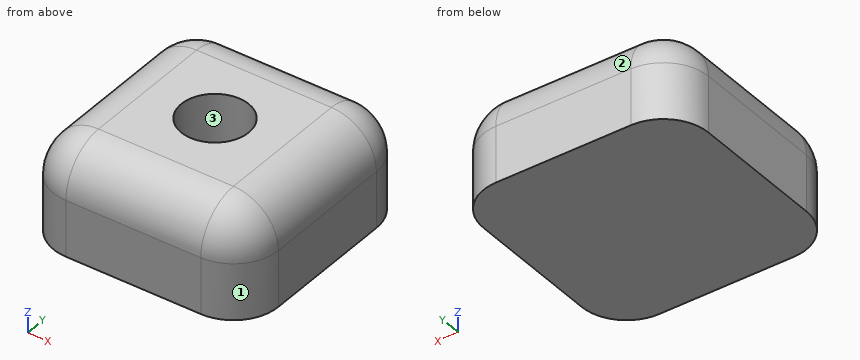
```python
from build123d import *

# Parameters (mm, degrees)
F0_W     = 25.4
F0_H     = 25.4
F1_DEPTH = 11.43
F2_R     = 3.81
F3_DEPTH = 6.35
F4_R     = 5.08


with BuildPart() as f1:
    # F0 (on Top) → F1 (new body)
    with BuildSketch(Plane.XY):
        with Locations((12.7, 12.7)):
            Rectangle(F0_W, F0_H)
    extrude(amount=F1_DEPTH)

    # F2 (on face) → F3 (cut)
    with BuildSketch(Plane.XY.offset(11.43)):
        with Locations((12.7, 12.7)):
            Circle(F2_R)
    extrude(amount=-F3_DEPTH, mode=Mode.SUBTRACT)

    # F4
    f4_edges = [f1.edges().sort_by_distance(p)[0] for p in [
        (25.4, 12.7, 11.43),
        (12.7, 25.4, 11.43),
        (0, 12.7, 11.43),
        (12.7, 0, 11.43),
        (25.4, 25.4, 5.715),
        (25.4, 0, 5.715),
        (0, 25.4, 5.715),
        (0, 0, 5.715),
    ]]
    fillet(f4_edges, radius=F4_R)


solid = f1.part
```
The listing builds one solid part. Answer for the finished solid, in the listing's coordinates (mm). Face numbers are marked on the shaded views. Coordinates: 2 decimals unless noted, no trailing zeros. Loops run counter-clockwise (first coordinate to the right, second up) from the corner with the lowest first, then second, coordinate; pieces in that order, holes last. Notation, with made-up numbers: (23.25, 31.25) -> (52.25, 31.25) arc R24 cw to (52.25, 62.25) -> close; hole circle Ø2 at (51.5, 63.5). An arc over 180 degrees is marked (long way). Use one line per item in the form item = value. Start each with the question number.
Item 1: The part is cut by section B-B on x = 12.7. Determine the outline of the cut face in (y, z).
Item 2: The part is cut by section A-A on z = 2.75. Determine the outline of the cut face in (x, y), then the cut area to 3 significant figures.
Item 3: The mould has two halves that part along X. Classify the marked faces 1, 2 and 3: released by +X, released by -X, zero draft, split by the parting line, or undercut.
Item 4: Consider L1, parallel to Y at x = 12.7, z = 9.5; L2, parallel to Z at x = 14, y = 14.75; L3, parallel to Y at x = 12.7, z = 10. Determine where each line is inside the solid, lowest interval first. Write a range as [from, to].
Item 5: The part is cut by section D-D on z = 9.75. Determine the outline of the cut face in (x, y).
Item 6: A flat-ended cylindrical pin translates along its axis: pin 1 Ø1 at (y, z) = (16, 7) entering from -X. Find the tip coordinate at first contact, or state that the pin passes through.
Answer key:
q1.outline = (0, 0) -> (25.4, 0) -> (25.4, 6.35) arc R5.08 ccw to (20.32, 11.43) -> (16.51, 11.43) -> (16.51, 5.08) -> (8.89, 5.08) -> (8.89, 11.43) -> (5.08, 11.43) arc R5.08 ccw to (0, 6.35) -> close
q2.outline = (0, 5.08) arc R5.08 ccw to (5.08, 0) -> (20.32, 0) arc R5.08 ccw to (25.4, 5.08) -> (25.4, 20.32) arc R5.08 ccw to (20.32, 25.4) -> (5.08, 25.4) arc R5.08 ccw to (0, 20.32) -> close
q2.area = 623 mm2
q3.face_1 = released by +X
q3.face_2 = zero draft
q3.face_3 = undercut
q4.L1 = [1.09, 8.89], [16.51, 24.31]
q4.L2 = [0, 5.08]
q4.L3 = [1.55, 8.89], [16.51, 23.85]
q5.outline = (1.31, 5.08) arc R3.77 ccw to (5.08, 1.31) -> (20.32, 1.31) arc R3.77 ccw to (24.09, 5.08) -> (24.09, 20.32) arc R3.77 ccw to (20.32, 24.09) -> (5.08, 24.09) arc R3.77 ccw to (1.31, 20.32) -> close; hole circle Ø7.62 at (12.7, 12.7)
q6.pin_1 = 0
